```python
from build123d import *

# Parameters (mm, degrees)
SKETCH1_W           = 15
SKETCH1_H           = 15
BOSS_EXTRUDE1_DEPTH = 120
CUT_EXTRUDE1_DEPTH  = 110
CUT_EXTRUDE2_START  = -20.25
CUT_EXTRUDE2_DEPTH  = 1.5
LPATTERN1_COUNT     = 27
LPATTERN1_PITCH     = 3
CUT_EXTRUDE3_START  = -10
SKETCH6_W           = 7
SKETCH6_H           = 7
CUT_EXTRUDE3_DEPTH  = 5.5
CUT_EXTRUDE4_DEPTH  = 122.86057607


with BuildPart() as part:
    # Sketch1 → Boss-Extrude1 (new body)
    with BuildSketch(Plane(origin=(0, 0, 0), x_dir=(1, 0, 0), z_dir=(0, 1, 0))):
        with Locations((7.5, 7.5)):
            Rectangle(SKETCH1_W, SKETCH1_H)
    extrude(amount=BOSS_EXTRUDE1_DEPTH)

    # Sketch3 → Cut-Extrude1 (cut)
    with BuildSketch(Plane(origin=(0, 120, 0), x_dir=(1, 0, 0), z_dir=(0, 1, 0))):
        Polygon((15, 3), (13, 3), (13, 2), (11, 2), (11, 7.5), (13, 7.5), (13, 6.5), (15, 6.5), align=None)
        Polygon((3, 13), (2, 13), (2, 11), (7.5, 11), (7.5, 13), (6.5, 13), (6.5, 15), (3, 15), align=None)
    extrude(amount=-CUT_EXTRUDE1_DEPTH, mode=Mode.SUBTRACT)

    # Sketch5 → Cut-Extrude2 (cut)
    with BuildSketch(Plane(origin=(0, 120, 0), x_dir=(1, 0, 0), z_dir=(0, 1, 0)).offset(CUT_EXTRUDE2_START)):
        Polygon((15, 15), (15, 9.5), (9.5, 15), align=None)
    cut_extrude2 = extrude(amount=-CUT_EXTRUDE2_DEPTH, mode=Mode.SUBTRACT)

    # LPattern1: Cut-Extrude2 ×27
    with Locations(*[(0, -i * LPATTERN1_PITCH, 0) for i in range(1, LPATTERN1_COUNT)]):
        add(cut_extrude2, mode=Mode.SUBTRACT)

    # Sketch6 → Cut-Extrude3 (cut)
    with BuildSketch(Plane.XZ.offset(CUT_EXTRUDE3_START)):
        with Locations((11.5, -11.5)):
            Rectangle(SKETCH6_W, SKETCH6_H)
    extrude(amount=-CUT_EXTRUDE3_DEPTH, mode=Mode.SUBTRACT)

    # Sketch12 → Cut-Extrude4 (cut, through all)
    with BuildSketch(Plane.XY):
        with BuildLine():
            Line((0, 120), (15, 120))
            Line((15, 120), (15, 105))
            ThreePointArc((15, 105), (10.606601718, 115.606601718), (0, 120))
        make_face()
    extrude(amount=-CUT_EXTRUDE4_DEPTH, mode=Mode.SUBTRACT)


solid = part.part
```
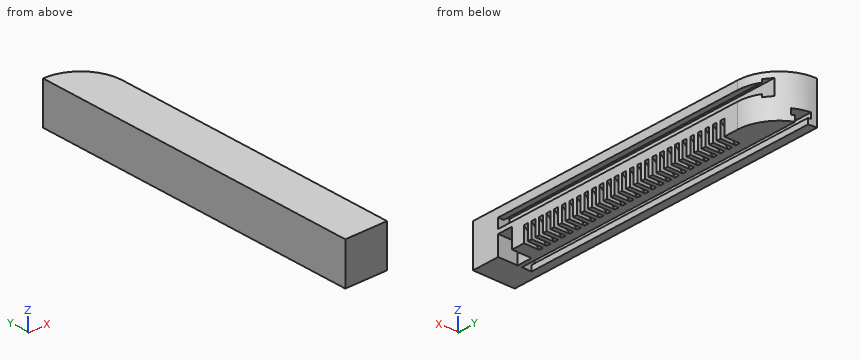
Verification items for the finished model (mm, model axes). Coordinates: 2 decimals unless noted, no trailing zeros. Write each loop counter-clockwise with the first axis right and the second up, starting at its lowest first coordinate (ties: lowest second). Pieces come first, ordered by that corner, then holes. Notation, with made-up numbers: M 1.25,-36.75 L 55.25,-36.75 A22 ccw 55.25,-15.75 Z; hole C -10.5,46 d4. An arc over 180 degrees is marked long. Answer as a JSON object with one key per item and string values. Group by question number.
(1) Gauge pin test, flat ends, axial feed: pin 1 (3 mm diameter, centred on x = 13.5, z = -13.5, fed in from -Y); pin 2 (3 mm diameter, centred on x = 11, z = -11.5, fed in from +Y); pin 3 (1 mm diameter, centred on y = 42, z = -13, fed in from +X); pin 4 (5.5 mm diameter, centred on x = 12, z = -12.5, fed in from +Y). Record the tip position at first contact, or that the pin passes through.
(2) Cross-section at A-A, the plane x = 4. Record the cut outline in (y, z).
(3) Cross-section at C-C, the plane z = -4. Record the cut outline in (x, y).
(4) Material ranges on line 1 (X direction, y = 49, z = -2.5); line 2 (Z direction, x = 2.5, y = 70); line 3 (Y direction, x = 12.5, z = -3.5), recorded low to high.
(5) Cross-section at B-B, the plane y = 107.5. Record the cut outline in (x, z), and give its area (3 significant figures).
Reply:
{
 "1": {"pin 1": "y = 0", "pin 2": "y = 116.61", "pin 3": "x = 12", "pin 4": "y = 116.81"},
 "2": {"outline": "M 0,-15 L 10,-15 L 10,-11 L 119.46,-11 L 119.46,0 L 0,0 Z"},
 "3": {"outline": "M 0,0 L 15,0 L 15,10 L 11,10 L 11,115.2 A15 ccw 0,120 Z"},
 "4": {"line 1": "0 to 11, 13 to 15", "line 2": "-15 to -13, -11 to 0", "line 3": "0 to 10"},
 "5": {"outline": "M 0,-15 L 3,-15 L 3,-13 L 2,-13 L 2,-11 L 7.5,-11 L 7.5,-13 L 6.5,-13 L 6.5,-15 L 14.79,-15 L 14.79,-6.5 L 13,-6.5 L 13,-7.5 L 11,-7.5 L 11,-2 L 13,-2 L 13,-3 L 14.79,-3 L 14.79,0 L 0,0 Z", "area": "187 mm²"}
}
